The model under review builds one solid part; all positions refer to its coordinate system, in mm. A direction names the side the tool comes from. Give positions to 0.01 mm unless a question says otherwise; leave off trailing zeros. Loops run counter-clockwise (first coordinate to the right, second up) from the corner with the lowest first, then second, coordinate; pieces in that order, holes last. Notation, with made-up numbers: (-11.5, -30) -> (29.5, -30) arc R22 cw to (29.5, -24) -> close; hole circle Ø8 at (72, 82). An arc over 180 degrees is marked (long way). Write each question's results on one line, items separated by ' | '. Start each with the question number.
Q1. Machinability: for faces 4 (the face through (27.232, 1.562, 0.105)), 5 (the face through (13.17, -0.01, -5.12)), which of the approach directions +Z, -Z, +X, -X, +Y, -Y give a long, thin tool a straight path to every point of the face, cutting with its end or side? Answer none if there is none.
Q2. Wall thickness on L1, parallel to X at y = 3, z = 6.25; L2, parallel to Y at x = 20.75, z = 3; L3, parallel to Z at x = 22, y = -0.5: over which ranges is each line inside the solid? List them lowest first. Write a range as [from, to].
Q3. Mouldability with a two-part tool opening along Y and no side actions: class faces 1 (the face through (4.93, -0.07, -1.5)), 2 (the face through (20.09, -0.737, -1.894)), 3 (the face through (0, 0, 0)) as released by +Y, released by -Y, zero draft, split by the parting line, or undercut.
Q4. We need section C-C (z = 6.75). Write out the cut boundary in (x, y), plus the area to 3 significant figures.
Q5. Insertion check: pin 1 Ø1.5 at (x, y) = (22.5, 3) entering from +Z; pin 2 Ø6 at (x, y) = (16.5, 5.5) entering from -Z; pin 3 Ø1.5 at (x, z) = (22, -3) entering from -Y. Each pin has a flat end and moves straight along its axis. Give the tip position at first contact, or say it passes through.
Q6. We need section A-A (x = 5.5). Write out the cut boundary in (y, z), plus the area to 3 significant figures.
Q7. We need section B-B (y = 0). Write out the cut boundary in (x, z), plus the area to 3 significant figures.
Q8. We need section D-D (y = 4.5). Write out the cut boundary in (x, z).
from build123d import *

# Parameters (mm, degrees)
F3_DEPTH      = 7.501
F3_DEPTH_BACK = 7.501
F4_R          = 1
F5_DEPTH      = 15


with BuildPart() as f1:
    # F0 (on Front) → F1 (revolve)
    with BuildSketch(Plane.XZ):
        Polygon((30, 7.5), (10, 7.5), (10, 1.5), (0, 1.5), (0, 0), (30, 0), align=None)
    revolve(axis=Axis((8.7773360142, 0, 0), (1, 0, 0)))

    # F2 (on Front) → F3 (cut, two sides)
    with BuildSketch(Plane.XZ) as f3_sk:
        Polygon((24.540446486, 7.5), (30, -7.5), (30, 7.5), align=None)
    extrude(amount=-F3_DEPTH, mode=Mode.SUBTRACT)
    extrude(f3_sk.sketch, amount=F3_DEPTH_BACK, mode=Mode.SUBTRACT)

    # F4 (on face) → F5 (cut)
    with BuildSketch(Plane(origin=(24.0802131105, 0, 8.764480807), x_dir=(0, 1, 0), z_dir=(0.9396926208, 0, 0.3420201433))):
        with Locations((0, -9.3269656621)):
            Circle(F4_R)
    extrude(amount=-F5_DEPTH, mode=Mode.SUBTRACT)


solid = f1.part
Output:
1) face 4: +Z, +X, +Y, -Y | face 5: none
2) L1: [10, 25] | L2: [-6.87, 6.87] | L3: [-7.48, -2.84], [-1, 7.48]
3) face 1: split by the parting line | face 2: undercut | face 3: zero draft
4) outline: (10, -3.27) -> (24.81, -3.27) -> (24.81, 3.27) -> (10, 3.27) -> close | area: 96.9 mm2
5) pin 1: z = 7.15 | pin 2: z = -7.07 | pin 3: y = -7.15
6) outline: circle Ø3 at (0, 0) | area: 7.07 mm2
7) outline: (0, -1.5) -> (10, -1.5) -> (10, -7.5) -> (30, -7.5) -> (27.61, -0.94) -> (13.52, -6.07) -> (12.83, -4.19) -> (26.93, 0.94) -> (24.54, 7.5) -> (10, 7.5) -> (10, 1.5) -> (0, 1.5) -> close | area: 259 mm2
8) outline: (10, -6) -> (29.45, -6) -> (25.09, 6) -> (10, 6) -> close
